Input: part model. Units: mm. Frame: model coordinates. A direction names the side the tool comes from. Round coordinates to 2 decimals unless told otherwise and drop trailing zeros. Loops run counter-clockwise (first coordinate to the right, second up) from the corner with the lowest first, then second, coordinate; pieces in that order, holes last. Notation, with made-up numbers: M -3.75,61 L 38.25,61 A24 cw 38.25,78 Z; hole C 73.25,84 d8. An arc over 180 degrees is marked long. Return JSON: item names as keys, results as strings. Group by question number.
1) Section D-D (y = -11.5). Output: boundary loops of the cut face in (x, z) (1 decimal).
2) Access query for faces 5 (the face through (24, 13.325, 1)), 6 (the face through (-26.127, -17.207, 0.783)). Directions: +Z, -Z, +X, -X, +Y, -Y. A direction counts if a zero-diameter tool reaches every point of the face in a straight line with its end or side. Return the directions, or none.
3) Material intervals for line 1 (Y direction, x = -24.13, z = 0.4); line 2 (X direction, y = -8.5, z = 0.8); line 3 (X direction, y = -7, z = 1.4), sorted ascending. Write a range as from..to.
4) Section A-A (x = 0). Output: boundary loops of the cut face in (y, z).
5) Contact query for a flat-ended pin moving along its axis: P1, Ø0.8, axis at x = -23.5, z = 0.5, coming from the -Y side. Output: stop coordinate, or through.
6) Section B-B (x = -24.13). Output: boundary loops of the cut face in (y, z), plus the area to 3 significant figures.
7) Section C-C (y = 15.24). Output: boundary loops of the cut face in (x, z).
8) Mould query, pull axis Y, two halves, no side actions, for faces 1 (the face through (-24, -10.424, 1)), 2 (the face through (0, 17.78, 1)), 3 (the face through (-1.84, -19.69, 0.78)), 4 (the face through (0, 3, 0)). Classes: +Y half, -Y half, draft (parallel to the pull), parting line (faces both ways), or undercut.
from build123d import *

# Parameters (mm, degrees)
SKETCH1_R           = 0.60325
BOSS_EXTRUDE1_DEPTH = 1.5875
SKETCH5_W           = 1.5875
SKETCH5_H           = 3.175
SKETCH5_H_2         = 4.699
CUT_EXTRUDE1_DEPTH  = 34.530212411
SKETCH7_R           = 1.3589
CUT_EXTRUDE2_DEPTH  = 34.530212411
SKETCH8_R           = 6.222246918
SKETCH8_R_2         = 4.114931659
CUT_EXTRUDE3_DEPTH  = 34.530212411
SKETCH9_R           = 2.787155445
CUT_EXTRUDE4_DEPTH  = 34.530212411


with BuildPart() as part:
    # Sketch1 → Boss-Extrude1 (new body)
    with BuildSketch(Plane.XY):
        with BuildLine():
            ThreePointArc((26.67, 15.875), (26.112038418, 17.222038418), (24.765, 17.78))
            Line((24.765, 17.78), (-24.765, 17.78))
            ThreePointArc((-24.765, 17.78), (-26.112038418, 17.222038418), (-26.67, 15.875))
            Line((-26.67, 15.875), (-26.67, -15.875))
            ThreePointArc((-26.67, -15.875), (-26.112038418, -17.222038418), (-24.765, -17.78))
            Line((-24.765, -17.78), (-7.62, -17.78))
            Line((-7.62, -17.78), (-2.103962754, -20.259962687))
            Line((-2.103962754, -20.259962687), (-1.567237562, -19.108951797))
            ThreePointArc((-1.567237562, -19.108951797), (0, -12.0396), (1.567237562, -19.108951797))
            Line((1.567237562, -19.108951797), (2.103962754, -20.259962687))
            Line((2.103962754, -20.259962687), (7.62, -17.78))
            Line((7.62, -17.78), (24.765, -17.78))
            ThreePointArc((24.765, -17.78), (26.112038418, -17.222038418), (26.67, -15.875))
            Line((26.67, -15.875), (26.67, 15.875))
        make_face()
        with Locations((-24.13, -15.24)):
            Circle(SKETCH1_R, mode=Mode.SUBTRACT)
        with Locations((24.13, -15.24)):
            Circle(SKETCH1_R, mode=Mode.SUBTRACT)
        with Locations((-24.13, 15.24)):
            Circle(SKETCH1_R, mode=Mode.SUBTRACT)
        with Locations((24.13, 15.24)):
            Circle(SKETCH1_R, mode=Mode.SUBTRACT)
    extrude(amount=BOSS_EXTRUDE1_DEPTH)

    # Sketch5 → Cut-Extrude1 (cut, through all)
    with BuildSketch(Plane.XY.offset(1.5875)):
        with Locations((23.97125, -12.011129894)):
            Rectangle(SKETCH5_W, SKETCH5_H)
        with Locations((23.97125, 10.975870106)):
            Rectangle(SKETCH5_W, SKETCH5_H_2)
    cut_extrude1 = extrude(amount=-CUT_EXTRUDE1_DEPTH, mode=Mode.SUBTRACT)

    # Mirror1: Cut-Extrude1 across plane
    add(cut_extrude1.mirror(Plane(origin=(0, 0, 0), x_dir=(0, 0, 1), z_dir=(1, 0, 0))), mode=Mode.SUBTRACT)

    # Sketch7 → Cut-Extrude2 (cut, through all)
    with BuildSketch(Plane.XY.offset(1.5875)):
        with Locations((0, 10.795)):
            Circle(SKETCH7_R)
        with Locations((9.5377, 2.8702)):
            Circle(SKETCH7_R)
        with Locations((-9.5377, 2.8702)):
            Circle(SKETCH7_R)
        with Locations((0, -5.0546)):
            Circle(SKETCH7_R)
    extrude(amount=-CUT_EXTRUDE2_DEPTH, mode=Mode.SUBTRACT)

    # Sketch8 → Cut-Extrude3 (cut, through all)
    with BuildSketch(Plane.XY.offset(1.5875)):
        with Locations(Location((13.780253082, -8.382753082, 0), (0, 0, 180))):
            Circle(SKETCH8_R)
        with Locations((-15.887568341, 10.490068341)):
            Circle(SKETCH8_R_2)
        with Locations((-13.780253082, -8.382753082)):
            Circle(SKETCH8_R)
        with Locations(Location((15.887568341, 10.490068341, 0), (0, 0, 180))):
            Circle(SKETCH8_R_2)
    extrude(amount=-CUT_EXTRUDE3_DEPTH, mode=Mode.SUBTRACT)

    # Sketch9 → Cut-Extrude4 (cut, through all)
    with BuildSketch(Plane.XY.offset(1.5875)):
        with Locations((-20.707844555, 1.640626454)):
            Circle(SKETCH9_R)
        with Locations(Location((20.707844555, 1.640626454, 0), (0, 0, 180))):
            Circle(SKETCH9_R)
    extrude(amount=-CUT_EXTRUDE4_DEPTH, mode=Mode.SUBTRACT)


solid = part.part
Returned:
{
 "1": {"outline": "M -26.7,0 L -24.8,0 L -24.8,1.6 L -26.7,1.6 Z; M -23.2,0 L -19.2,0 L -19.2,1.6 L -23.2,1.6 Z; M -8.4,0 L 8.4,0 L 8.4,1.6 L -8.4,1.6 Z; M 19.2,0 L 23.2,0 L 23.2,1.6 L 19.2,1.6 Z; M 24.8,0 L 26.7,0 L 26.7,1.6 L 24.8,1.6 Z"},
 "2": {"face 5": "+Z, -Z", "face 6": "+Z, -Z, -X, -Y"},
 "3": {"line 1": "y = -17.78..-15.84, -14.64..-13.6, -10.42..8.63, 13.33..14.64, 15.84..17.78", "line 2": "x = -26.67..-20, -7.56..7.56, 20..26.67", "line 3": "x = -26.67..-19.85, -7.71..7.71, 19.85..26.67"},
 "4": {"outline": "M -12.04,0 L -6.41,0 L -6.41,1.59 L -12.04,1.59 Z; M -3.7,0 L 9.44,0 L 9.44,1.59 L -3.7,1.59 Z; M 12.15,0 L 17.78,0 L 17.78,1.59 L 12.15,1.59 Z"},
 "5": {"P1": "stops at y = -17.78"},
 "6": {"outline": "M -17.78,0 L -15.84,0 L -15.84,1.59 L -17.78,1.59 Z; M -14.64,0 L -13.6,0 L -13.6,1.59 L -14.64,1.59 Z; M -10.42,0 L 8.63,0 L 8.63,1.59 L -10.42,1.59 Z; M 13.33,0 L 14.64,0 L 14.64,1.59 L 13.33,1.59 Z; M 15.84,0 L 17.78,0 L 17.78,1.59 L 15.84,1.59 Z", "area": "40.1 mm^2"},
 "7": {"outline": "M -26.67,0 L -24.73,0 L -24.73,1.59 L -26.67,1.59 Z; M -23.53,0 L 23.53,0 L 23.53,1.59 L -23.53,1.59 Z; M 24.73,0 L 26.67,0 L 26.67,1.59 L 24.73,1.59 Z"},
 "8": {"face 1": "undercut", "face 2": "+Y half", "face 3": "-Y half", "face 4": "draft"}
}
